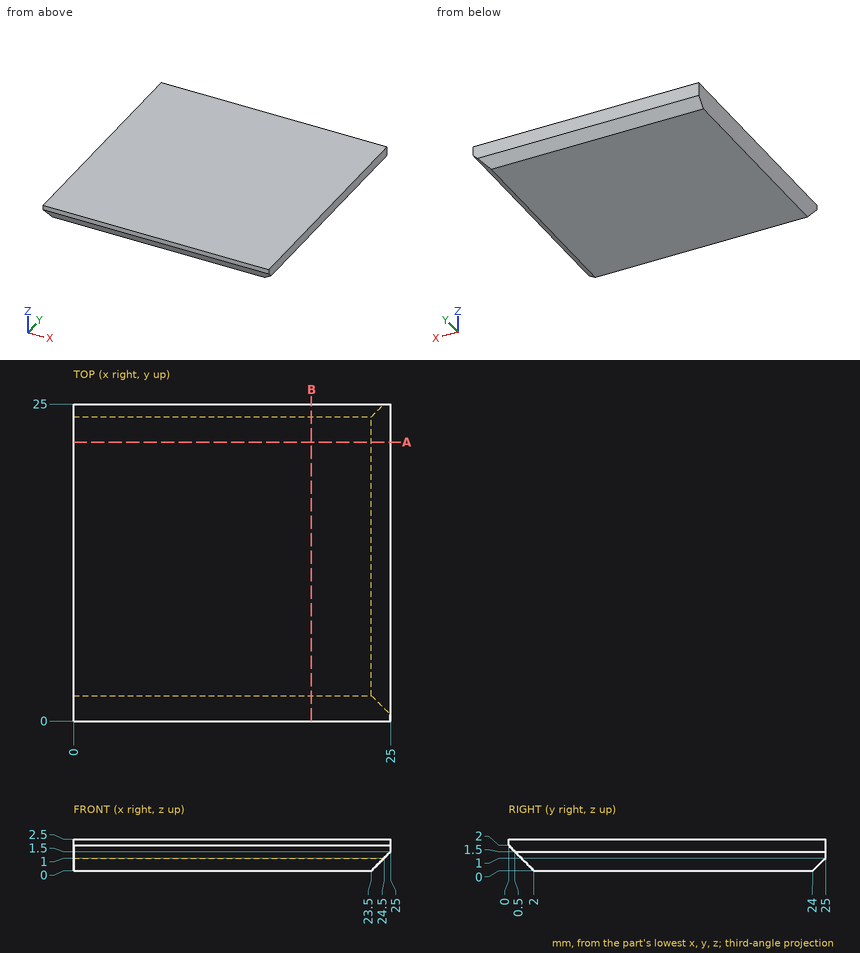
Here's the drawing with two shaded views (mm, measured from the low corner). I have some questions. Coordinates: 2 decimals unless noted, no trailing zeros. Loops run counter-clockwise (first coordinate to the right, second up) from the corner with the lowest first, then second, coordinate; pieces in that order, holes last. Notation, with made-up numbers: (28.5, -5) - (80.5, -5) arc R12 cw to (80.5, -1) - close; hole circle Ø10 at (-27, -19). An arc over 180 degrees is marked (long way). Answer as CSV lines item,"result". Start each with the question number.
1) Suppose I cut it at A-A (y = 22). Please give me the cut outline in (x, z).
2) Suppose I cut it at B-B (x = 18.75). Please give me the cut outline in (y, z).
3) I need wall thicknesses on line 1 (Y direction, x = 20, z = 1.5); line 2 (X direction, y = 11, z = 0.8); line 3 (Y direction, x = 2.25, z = 0.35). Which ranges of each line are inside material? Lowest first, please. Write a range as from..to.
Check result:
1,outline,"(0, 0) - (23.5, 0) - (25, 1.5) - (25, 2.5) - (0, 2.5) - close"
2,outline,"(0, 2) - (2, 0) - (24, 0) - (25, 1) - (25, 2.5) - (0, 2.5) - close"
3,line 1,"y = 0.5..25"
3,line 2,"x = 0..24.3"
3,line 3,"y = 1.65..24.35"
